```python
from build123d import *

# Parameters (mm, degrees)
F0_W     = 3.048
F0_H     = 5.842
F2_DEPTH = 3.81
F3_SIZE  = 0.508


with BuildPart() as f1:
    # F0 (on Front) → F1 (revolve)
    with BuildSketch(Plane.XZ):
        Polygon((0, 9.652), (0, 5.842), (3.2385, 5.842), (3.2385, 0), (5.08, 0), (5.08, -3.048), (8.255, -3.048), (8.255, 9.652), align=None)
    revolve(axis=Axis((0, 0, 7.747), (0, 0, -1)))

    # F0 (on Front) → F2 (join, symmetric)
    with BuildSketch(Plane.XZ):
        with Locations((-2.9845, 3.1697918537)):
            Rectangle(F0_W, F0_H)
    extrude(amount=F2_DEPTH, both=True)

    # F3
    f3_edges = [f1.edges().sort_by_distance(p)[0] for p in [
        (-8.255, 0, 9.652),
    ]]
    chamfer(f3_edges, length=F3_SIZE)


solid = f1.part
```
The listing builds one solid part. Answer for the finished solid, in the listing's coordinates (mm). A direction names the side the tool comes from. Give positions to 0.01 mm unless a question says otherwise; leave off trailing zeros. Order: outer loops, then holes, each group sorted by start corner. A loop starts at its lowest first (then second) coordinate and runs counter-clockwise, first axis right, second up. Notation, with made-up numbers: (40.25, 71.5) -> (81.25, 71.5) arc R23 ccw to (81.25, 109.5) -> close; hole circle Ø1 at (-31.5, 0). An arc over 180 degrees is marked (long way). Answer as CSV lines item,"result". Start each with the question number.
Q1. Find the intervals of material crossed by L1, parallel to Y at x = 0, z = -1.45 (3 decimals); L2, parallel to Y at x = 0, z = 4.2 (1 decimal), in increasing order.
Q2. A cutting plane is placed at B-B (x = 0). Determine the outline of the cut face in (y, z) (1 decimal), then the cut area to 3 significant figures.
Q3. Which of the six approach directions +Z, -Z, +X, -X, +Y, -Y give full straight-line access (tool end or side, diameter ignored) to faces 1 (the flat face through (-1.461, 0, 3)), 2 (the cylindrical face through (7.874, -2.48, 3.133))?
Q4. A cutting plane is placed at C-C (z = -2). Determine the outline of the cut face in (x, y) (3 decimals).
Q5. A cutting plane is placed at D-D (z = 7). Determine the outline of the cut face in (x, y) (3 decimals).
Q6. Given pin 1 (1 mm diameter, centred on x = 1, z = 0, fed in from -Y); pin 2 (5 mm diameter, centred on x = 1, y = 1, fed in from -Z); pin 3 (3 mm diameter, centred on y = -4, z = -1.5, fed in from +X), each flat-ended and moving along its own axis, determine where each tip first touches the part or whether it passes through.
Results found:
1,L1,"-8.255 to -5.08, 5.08 to 8.255"
1,L2,"-8.3 to -3.2, 3.2 to 8.3"
2,outline,"(-8.3, -3) -> (-5.1, -3) -> (-5.1, 0) -> (-3.2, 0) -> (-3.2, 5.8) -> (3.2, 5.8) -> (3.2, 0) -> (5.1, 0) -> (5.1, -3) -> (8.3, -3) -> (8.3, 9.1) -> (7.7, 9.7) -> (-7.7, 9.7) -> (-8.3, 9.1) -> close"
2,area,"141 mm2"
3,face 1,"-Z"
3,face 2,"+Z, -Z"
4,outline,"circle Ø16.51 at (0, 0); hole circle Ø10.16 at (0, 0)"
5,outline,"circle Ø16.51 at (0, 0)"
6,pin 1,"y = -8.24"
6,pin 2,"z = 0"
6,pin 3,"x = 7.87"
